Input: part model. Units: mm. Frame: model coordinates. A direction names the side the tool comes from. Round coordinates to 2 decimals unless told otherwise and drop trailing zeros. Order: outer loops, then holes, each group sorted by start corner. A loop starts at its lowest first (then second) coordinate and runs counter-clockwise, first axis right, second up. Notation, with made-up numbers: M 33.25,45 L 84.25,45 A15 ccw 84.25,68 Z; hole C 4,71.5 d5. An arc over 180 degrees is marked long. One line per question, with ' | ' between items.
```python
from build123d import *

# Parameters (mm, degrees)
SKETCH1_R             = 4.3
BOSS_EXTRUDE1_DEPTH   = 10
BOSS_EXTRUDE1_2_DEPTH = 10
BOSS_EXTRUDE1_3_DEPTH = 10
BOSS_EXTRUDE1_4_DEPTH = 10
SKETCH2_W             = 10
SKETCH2_H             = 9
BOSS_EXTRUDE2_DEPTH   = 80
SKETCH3_W             = 109
SKETCH3_H             = 58.5
BOSS_EXTRUDE3_DEPTH   = 5
FILLET1_R             = 15
SKETCH4_R             = 1.275
SKETCH4_R_2           = 6.75
CUT_EXTRUDE1_DEPTH    = 5


with BuildPart() as part:
    # Sketch1 → Boss-Extrude1 (new body)
    with BuildSketch(Plane(origin=(0, 0, 0), x_dir=(1, 0, 0), z_dir=(0, 1, 0))):
        with Locations(Location((49.5, 0, 0), (0, 0, 270))):
            Circle(SKETCH1_R)
    extrude(amount=BOSS_EXTRUDE1_DEPTH)



with BuildPart() as body_2:
    # Sketch1 → Boss-Extrude1 2 (new body)
    with BuildSketch(Plane(origin=(0, 0, 0), x_dir=(1, 0, 0), z_dir=(0, 1, 0))):
        with Locations(Location((-49.5, 0, 0), (0, 0, 90))):
            Circle(SKETCH1_R)
    extrude(amount=BOSS_EXTRUDE1_2_DEPTH)


with BuildPart() as body_3:
    # Sketch1 → Boss-Extrude1 3 (new body)
    with BuildSketch(Plane(origin=(0, 0, 0), x_dir=(1, 0, 0), z_dir=(0, 1, 0))):
        with Locations(Location((49.5, 49.5, 0), (0, 0, 270))):
            Circle(SKETCH1_R)
    extrude(amount=BOSS_EXTRUDE1_3_DEPTH)


with BuildPart() as body_4:
    # Sketch1 → Boss-Extrude1 4 (new body)
    with BuildSketch(Plane(origin=(0, 0, 0), x_dir=(1, 0, 0), z_dir=(0, 1, 0))):
        with Locations(Location((-49.5, 49.5, 0), (0, 0, 90))):
            Circle(SKETCH1_R)
    extrude(amount=BOSS_EXTRUDE1_4_DEPTH)


with BuildPart() as part_1:
    add(part.part)

    add(body_2.part)  # Boss-Extrude2 merges body 2

    add(body_3.part)  # Boss-Extrude2 merges body 3

    add(body_4.part)  # Boss-Extrude2 merges body 4
    # Sketch2 → Boss-Extrude2 (add)
    with BuildSketch(Plane(origin=(0, 10, 0), x_dir=(1, 0, 0), z_dir=(0, 1, 0))):
        with Locations((49.5, 0)):
            Rectangle(SKETCH2_W, SKETCH2_H)
        with Locations((-49.5, 0)):
            Rectangle(SKETCH2_W, SKETCH2_H)
        with Locations((49.5, 49.5)):
            Rectangle(SKETCH2_W, SKETCH2_H)
        with Locations((-49.5, 49.5)):
            Rectangle(SKETCH2_W, SKETCH2_H)
    extrude(amount=BOSS_EXTRUDE2_DEPTH)

    # Sketch3 → Boss-Extrude3 (add)
    with BuildSketch(Plane(origin=(0, 90, 0), x_dir=(1, 0, 0), z_dir=(0, 1, 0))):
        with Locations((0, 24.75)):
            Rectangle(SKETCH3_W, SKETCH3_H)
    extrude(amount=BOSS_EXTRUDE3_DEPTH)

    # Fillet1
    fillet1_edges = [part_1.edges().sort_by_distance(p)[0] for p in [
        (49.5, 90, -4.5),
        (44.5, 90, 0),
        (-44.5, 90, 0),
        (-49.5, 90, -4.5),
        (44.5, 90, -49.5),
        (49.5, 90, -45),
        (-44.5, 90, -49.5),
        (-49.5, 90, -45),
    ]]
    fillet(fillet1_edges, radius=FILLET1_R)

    # Sketch4 → Cut-Extrude1 (cut)
    with BuildSketch(Plane(origin=(0, 95, 0), x_dir=(1, 0, 0), z_dir=(0, 1, 0))):
        with Locations(Location((-0.965131435, 40.72196281, 0), (0, 0, 270))):
            Circle(SKETCH4_R)
        with Locations(Location((13.408900265, 17.47196281, 0), (0, 0, 270))):
            Circle(SKETCH4_R)
        with Locations(Location((-13.420367633, 16.50222878, 0), (0, 0, 270))):
            Circle(SKETCH4_R)
        with Locations(Location((0.003026126, 25.25222878, 0), (0, 0, 270))):
            Circle(SKETCH4_R_2)
    extrude(amount=-CUT_EXTRUDE1_DEPTH, mode=Mode.SUBTRACT)


solid = part_1.part
```
Item 1: Section query B-B, the plane z = -26. Return loops of the section in (x, y).
Report:
outline: M -54.5,90 L -6.71,90 L -6.71,95 L -54.5,95 Z; M 6.71,90 L 54.5,90 L 54.5,95 L 6.71,95 Z
Item 2: Section query D-D, the plane z = 0. Return loops of the section in (x, y), plus the area to 3 significant figures.
Report:
outline: M -54.5,10 L -53.8,10 L -53.8,0 L -45.2,0 L -45.2,10 L -44.5,10 L -44.5,75 A15 cw -29.5,90 L 29.5,90 A15 cw 44.5,75 L 44.5,10 L 45.2,10 L 45.2,0 L 53.8,0 L 53.8,10 L 54.5,10 L 54.5,95 L -54.5,95 Z | area: 2,410 mm²
Item 3: Mould query, pull axis X, two halves, no side actions, for faces 6 (the flat face through (-54, 10, 0)), 7 (the flat face through (50, 0, -50)), 8 (the cylindrical face through (-45.685, 4.93, -51.484)). Classes: +X half, -X half, draft (parallel to the pull), parting line (faces both ways), or undercut.
Report:
face 6: undercut | face 7: draft | face 8: undercut
Item 4: Access query for faces 1 (the cylindrical face through (38.24, 87.19, -44.83)), 2 (the flat face through (-4, 93, -54)), 3 (the cylindrical face through (44.95, 87.19, -10.76)), 4 (the cylindrical face through (45.685, 4.93, -47.516)), 5 (the cylindrical face through (13.792, 92.535, -16.256)). Directions: +Z, -Z, +X, -X, +Y, -Y. A direction counts if a zero-diameter tool reaches every point of the face in a straight line with its end or side. Return the directions, or none.
Report:
face 1: +Z, -Z, -Y | face 2: -Z, +X, -X, +Y, -Y | face 3: +X, -X, -Y | face 4: -Y | face 5: +Y, -Y
Item 5: Line query: line 1 along Y through (x, z) = (26, -12); line 2 along X through (y, z) = (34, -4); line 3 along Y through (x, z) = (-33, -44). Output: solid intervals per line, ascending. Write a range as from..to.
Report:
line 1: 90..95 | line 2: -54.5..-44.5, 44.5..54.5 | line 3: 89.59..95
Item 6: First-contact query: pin 1 (3.5 mm diameter, centred on x = -0.97, z = -40.72, fed in from -Y); pin 2 (4 mm diameter, centred on x = -38.5, z = -43.5, fed in from -Y); pin 3 (11 mm diameter, centred on x = 0, z = -25.25, fed in from +Y). Flat tips, straight axial feed; report the tip coordinate or a pass-through.
Report:
pin 1: y = 90 | pin 2: y = 85.2 | pin 3: through
Item 7: Section query A-A, the plane y = 20. Return loops of the section in (x, z), plus the area to 3 significant figures.
Report:
outline: M -54.5,-54 L -44.5,-54 L -44.5,-45 L -54.5,-45 Z; M -54.5,-4.5 L -44.5,-4.5 L -44.5,4.5 L -54.5,4.5 Z; M 44.5,-54 L 54.5,-54 L 54.5,-45 L 44.5,-45 Z; M 44.5,-4.5 L 54.5,-4.5 L 54.5,4.5 L 44.5,4.5 Z | area: 360 mm²
Item 8: Section query C-C, the plane x = 49.5. Return loops of the section in (y, z).
Report:
outline: M 0,-53.8 L 10,-53.8 L 10,-54 L 95,-54 L 95,4.5 L 10,4.5 L 10,4.3 L 0,4.3 L 0,-4.3 L 10,-4.3 L 10,-4.5 L 75,-4.5 A15 cw 90,-19.5 L 90,-30 A15 cw 75,-45 L 10,-45 L 10,-45.2 L 0,-45.2 Z
